Input: part model. Units: mm. Frame: model coordinates. A direction names the side the tool comes from. Coordinates: 2 decimals unless noted, no trailing zeros. Loops run counter-clockwise (first coordinate to the right, second up) from the corner with the lowest first, then second, coordinate; pieces in that order, holes last.
(1) Contact query for flat-ended pins moving along their axis: P1, Ø3, axis at x = -62, y = 19, coming from the +Z side (3 decimals); P2, Ø4, axis at y = 5, z = 16, coming from the +X side; P3, Ø2, axis at y = 5, z = 12.5, coming from the -X side; P4, Ø7.5, axis at x = -387.35, z = 14.29, coming from the +Y side (3 decimals). Output: stop coordinate, or through.
(2) Section A-A, the plane x = -429. Return loops of the section in (y, z) (3 decimals), then the cut area to 3 significant figures.
(3) Section B-B, the plane y = 13.5. Return loops of the section in (x, z) (3 decimals), then the cut area to 3 significant figures.
(4) Line query: L1, parallel to Z at x = -146.05, y = 2.15; L2, parallel to Y at x = -479, z = 14.75 (3 decimals). Output: solid intervals per line, ascending.
(5) Set-up query: faces 1 (the face through (-258, 14, 3.175)), 2 (the face through (-7, 2, 7)). Return all of +Z, -Z, +X, -X, +Y, -Y with unobstructed straight access to the full face (end or side cutting, diameter ignored); none if empty.
```python
from build123d import *

# Parameters (mm, degrees)
SKETCH1_W           = 508
SKETCH1_H           = 25.4
BOSS_EXTRUDE1_DEPTH = 3.175
SKETCH2_W           = 508
SKETCH2_H           = 3.175
BOSS_EXTRUDE2_DEPTH = 22.225
CUT_EXTRUDE4_DEPTH  = 25.4
SKETCH6_R           = 3.175
CUT_EXTRUDE5_DEPTH  = 3.175
CUT_EXTRUDE6_DEPTH  = 25.4


with BuildPart() as part:
    # Sketch1 → Boss-Extrude1 (new body)
    with BuildSketch(Plane(origin=(0, 0, 0), x_dir=(1, 0, 0), z_dir=(0, 1, 0))):
        with Locations((-254, -12.7)):
            Rectangle(SKETCH1_W, SKETCH1_H)
    extrude(amount=BOSS_EXTRUDE1_DEPTH)

    # Sketch2 → Boss-Extrude2 (add)
    with BuildSketch(Plane(origin=(0, 3.175, 0), x_dir=(1, 0, 0), z_dir=(0, 1, 0))):
        with Locations((-254, -1.5875)):
            Rectangle(SKETCH2_W, SKETCH2_H)
    extrude(amount=BOSS_EXTRUDE2_DEPTH)

    # Sketch3 → Cut-Extrude4 (cut)
    with BuildSketch(Plane(origin=(0, 25.4, 0), x_dir=(1, 0, 0), z_dir=(0, 1, 0))):
        Polygon((0, 0), (-52.33160776, -52.33160776), (49.536132654, -29.784007044), align=None)
    extrude(amount=-CUT_EXTRUDE4_DEPTH, mode=Mode.SUBTRACT)

    # Sketch6 → Cut-Extrude5 (cut)
    with BuildSketch(Plane(origin=(0, 3.175, 0), x_dir=(1, 0, 0), z_dir=(0, 1, 0))):
        with Locations((-146.05, -14.2875)):
            Circle(SKETCH6_R)
        with Locations((-387.35, -14.2875)):
            Circle(SKETCH6_R)
    extrude(amount=-CUT_EXTRUDE5_DEPTH, mode=Mode.SUBTRACT)

    # Sketch7 → Cut-Extrude6 (cut)
    with BuildSketch(Plane(origin=(0, 25.4, 0), x_dir=(1, 0, 0), z_dir=(0, 1, 0))):
        Polygon((-508, 0), (-469.606769631, -38.393230369), (-537.121608827, -29.121608827), align=None)
    extrude(amount=-CUT_EXTRUDE6_DEPTH, mode=Mode.SUBTRACT)


solid = part.part
```
Report:
1. P1: stops at z = 3.175
1. P2: stops at x = -15.18
1. P3: passes through
1. P4: stops at y = 3.175
2. outline: (0, 0) - (25.4, 0) - (25.4, 3.175) - (3.175, 3.175) - (3.175, 25.4) - (0, 25.4) - close
2. area: 151 mm2
3. outline: (-508, 0) - (0, 0) - (-3.175, 3.175) - (-504.825, 3.175) - close
3. area: 1,600 mm2
4. L1: z = 0 to 11.11, 17.46 to 25.4
4. L2: y = 0 to 3.175
5. face 1: +Z, +X, -X, +Y
5. face 2: +Z, +X, +Y, -Y
